Geometry: final body of the model. Coordinates: model frame, mm. A direction names the side the tool comes from. Give positions to 0.01 mm unless a question says otherwise; leave off trailing zeros. Loops run counter-clockwise (first coordinate to the right, second up) from the corner with the lowest first, then second, coordinate; pieces in that order, holes last.
from build123d import *

# Parameters (mm, degrees)
F0_R     = 2.25
F0_R_2   = 4.5
F0_R_3   = 6
F1_DEPTH = 15
F2_W     = 135
F2_H     = 4
F3_DEPTH = 20
F4_R     = 10


with BuildPart() as f1:
    # F0 (on Top) → F1 (new body)
    with BuildSketch(Plane.XY):
        with BuildLine():
            ThreePointArc((0, 8), (2.343146, 2.343146), (8, 0))
            Line((8, 0), (130, 0))
            ThreePointArc((130, 0), (172.36068, 3.81966), (150, 40))
            Line((150, 40), (0, 40))
            Line((0, 40), (0, 8))
        make_face()
        with Locations((10, 8)):
            Circle(F0_R, mode=Mode.SUBTRACT)
        with Locations((40, 8)):
            Circle(F0_R, mode=Mode.SUBTRACT)
        with Locations((70, 8)):
            Circle(F0_R, mode=Mode.SUBTRACT)
        with Locations((144.185658, -0.974775)):
            Circle(F0_R_2, mode=Mode.SUBTRACT)
        with Locations((158.5, 0.277568)):
            Circle(F0_R_2, mode=Mode.SUBTRACT)
        with Locations((100, 8)):
            Circle(F0_R, mode=Mode.SUBTRACT)
        with Locations((130, 8)):
            Circle(F0_R, mode=Mode.SUBTRACT)
        with Locations((166.741732, 12.047981)):
            Circle(F0_R_2, mode=Mode.SUBTRACT)
        with Locations((10, 25)):
            Circle(F0_R, mode=Mode.SUBTRACT)
        with Locations((40, 25)):
            Circle(F0_R, mode=Mode.SUBTRACT)
        with Locations((70, 25)):
            Circle(F0_R, mode=Mode.SUBTRACT)
        with Locations((100, 25)):
            Circle(F0_R, mode=Mode.SUBTRACT)
        with Locations((130, 25)):
            Circle(F0_R, mode=Mode.SUBTRACT)
        with Locations((150, 15)):
            Circle(F0_R_3, mode=Mode.SUBTRACT)
        with Locations((163.022756, 25.927389)):
            Circle(F0_R_2, mode=Mode.SUBTRACT)
        with Locations((150, 32)):
            Circle(F0_R_2, mode=Mode.SUBTRACT)
    extrude(amount=F1_DEPTH)

    # F2 (on face) → F3 (join)
    with BuildSketch(Plane.XY.offset(15)):
        with Locations((67.5, 38)):
            Rectangle(F2_W, F2_H)
    extrude(amount=F3_DEPTH)

    # F4
    f4_edges = [f1.edges().sort_by_distance(p)[0] for p in [
        (135, 38, 35),
        (0, 38, 35),
    ]]
    fillet(f4_edges, radius=F4_R)


solid = f1.part
Item 1: Set-up query: faces 4 (the face through (67, 36, 25)), 5 (the face through (167.18, 24.2, 7.4)). Return all of +Z, -Z, +X, -X, +Y, -Y with unobstructed straight access to the full face (end or side cutting, diameter ignored); none if empty.
Values follow:
face 4: +Z, +X, -X, -Y
face 5: +Z, -Z
Item 2: Section query B-B on y = 15. Return loops of the section in (x, z).
Values follow:
outline: (0, 0) - (144, 0) - (144, 15) - (0, 15) - close; (156, 0) - (163.35, 0) - (163.35, 15) - (156, 15) - close; (170.14, 0) - (175, 0) - (175, 15) - (170.14, 15) - close
Item 3: Section query D-D on x = 141.5. Return loops of the section in (y, z), plus the area to 3 significant figures.
Values follow:
outline: (-8.51, 0) - (-4.59, 0) - (-4.59, 15) - (-8.51, 15) - close; (2.64, 0) - (40, 0) - (40, 15) - (2.64, 15) - close
area: 619 mm2
Item 4: Ray query, probe 1 along Y at (x, z) = (100, 4.5); probe 2 along Z at (x, y) = (43, 34.5); probe 3 along Y at (x, z) = (113.5, 27). Return the intervals inside material, ascending.
Values follow:
probe 1: y = 0 to 5.75, 10.25 to 22.75, 27.25 to 40
probe 2: z = 0 to 15
probe 3: y = 36 to 40
Item 5: Section query A-A on x = 40. Return loops of the section in (y, z), plus the area to 3 significant figures.
Values follow:
outline: (0, 0) - (5.75, 0) - (5.75, 15) - (0, 15) - close; (10.25, 0) - (22.75, 0) - (22.75, 15) - (10.25, 15) - close; (27.25, 0) - (40, 0) - (40, 35) - (36, 35) - (36, 15) - (27.25, 15) - close
area: 545 mm2
Item 6: Draft query along X for faces 1 (the face through (0, 24, 7)), 2 (the face through (132.15, 38.03, 31.99)), 3 (the face through (39.512, 22.804, 7.395)). Return one class per face: +X half, -X half, draft (parallel to the pull), parting line (faces both ways), or undercut.
Values follow:
face 1: -X half
face 2: +X half
face 3: undercut
Item 7: Section query C-C on z = 13.5. Give the number of separate pieces and of enclosed holes in the cut face, plus the area to 3 significant figures.
Values follow:
separate pieces: 1
enclosed holes: 16
area: 6,520 mm2
Item 8: Pin query (flat end, axial travel): pin 1 (14.5 mm diameter, centred on x = 163.02, y = 25.93, fed in from -Z); pin 2 (16.5 mm diameter, centred on x = 42, z = 5.5, fed in from -Y); pin 3 (6 mm diameter, centred on x = 61, z = 23, fed in from -Y); pin 4 (5 mm diameter, centred on x = 10, y = 8, fed in from +Z). Return the tip coordinate at first contact, or that it passes through.
Values follow:
pin 1: stops at z = 0
pin 2: stops at y = 0
pin 3: stops at y = 36
pin 4: stops at z = 15
